```python
from build123d import *

# Parameters (mm, degrees)
SKETCH1_W            = 55
SKETCH1_H            = 164.75
BOSS_EXTRUDE1_DEPTH  = 6
M3_CLEARANCE_SLOT1_D = 3.2
SKETCH4_W            = 55
SKETCH4_H            = 6
BOSS_EXTRUDE2_DEPTH  = 6


with BuildPart() as part:
    # Sketch1 → Boss-Extrude1 (new body)
    with BuildSketch(Plane.XY):
        with Locations((27.5, 82.375)):
            Rectangle(SKETCH1_W, SKETCH1_H)
    extrude(amount=BOSS_EXTRUDE1_DEPTH)

    # M3 Clearance Slot1 (through all)
    with Locations(Plane(origin=(0, 0, 0), x_dir=(-1, 0, 0), z_dir=(0, 0, -1))):
        with Locations((-27.5, 161.67), (-27.5, 6.48)):
            Hole(M3_CLEARANCE_SLOT1_D / 2)

    # Sketch4 → Boss-Extrude2 (add)
    with BuildSketch(Plane(origin=(0, 164.75, 0), x_dir=(1, 0, 0), z_dir=(0, 1, 0))):
        with Locations((27.5, -3)):
            Rectangle(SKETCH4_W, SKETCH4_H)
    extrude(amount=BOSS_EXTRUDE2_DEPTH)


solid = part.part
```
Here's how the part is built. I have some questions about the finished solid (model axes, mm). Give positions to 0.01 mm unless a question says otherwise; leave off trailing zeros. Write each loop counter-clockwise with the first axis right and the second up, starting at its lowest first coordinate (ties: lowest second). Pieces come first, ordered by that corner, then holes. Notation, with made-up numbers: M 13,37 L 54,37 A6 cw 54,46 Z; hole C -9,36 d6. An arc over 180 degrees is marked long. Put each result on its own line as item: value. Start each with the question number.
Item 1: Will this pin go through, and if not, where does the flat tip stop? pin 1 (3 mm diameter, centred on x = 27.5, y = 161.67, fed in from +Z).
Item 2: If we section it at B-B, the plane x = 27.5: Write out the boundary of the cut face in (y, z), then the cut area to 3 significant figures.
Item 3: Thinking about a two-plate mould opening in Y: for faces 1 (the cylindrical face through (26.23, 5.51, 3.04)), 2 (the flat face through (27, 170.75, 3)), 3 (the flat face through (27, 84, 0)), which applies, +Y half, -Y half, draft (parallel to the pull), parting line (faces both ways), or undercut?
Item 4: If we section it at A-A, the plane y = 161.67: Write out the boundary of the cut face in (x, z).
Item 5: I need wall thicknesses on L1, parallel to Y at x = 27.5, z = 1.5; L2, parallel to X at y = 161.67, z = 1.6; L3, parallel to Y at x = 26.5, z = 4.4. Which ranges of each line are inside material? Lowest first, please. Write a range as from..to.
Values:
1. pin 1: through
2. outline: M 0,0 L 4.88,0 L 4.88,6 L 0,6 Z; M 8.08,0 L 160.07,0 L 160.07,6 L 8.08,6 Z; M 163.27,0 L 170.75,0 L 170.75,6 L 163.27,6 Z
2. area: 986 mm²
3. face 1: undercut
3. face 2: +Y half
3. face 3: draft
4. outline: M 0,0 L 25.9,0 L 25.9,6 L 0,6 Z; M 29.1,0 L 55,0 L 55,6 L 29.1,6 Z
5. L1: 0..4.88, 8.08..160.07, 163.27..170.75
5. L2: 0..25.9, 29.1..55
5. L3: 0..5.23, 7.73..160.42, 162.92..170.75
